Work out the finished part from the listing and answer in its coordinate system (mm). A direction names the side the tool comes from. Coordinates: 2 decimals unless noted, no trailing zeros. Order: outer loops, then holes, each group sorted by start corner. A loop starts at its lowest first (then second) coordinate and runs counter-clockwise, first axis right, second up. Notation, with made-up numbers: M 3.5,0.5 L 39.5,0.5 A37 ccw 39.5,37.5 Z; hole C 72.5,-3 d7. An arc over 180 degrees is marked long. Use a Markdown table: item, result.
from build123d import *

# Parameters (mm, degrees)
SKETCH1_W                      = 15.75
SKETCH1_H                      = 21.4
BOSS_EXTRUDE1_DEPTH            = 12.7
SKETCH3_W                      = 0.75
SKETCH3_H                      = 4
SKETCH4_W                      = 0.75
SKETCH4_H                      = 4
SKETCH5_W                      = 0.75
SKETCH5_H                      = 4
SKETCH6_W                      = 0.75
SKETCH6_H                      = 4
SKETCH7_W                      = 0.75
SKETCH7_H                      = 4
SKETCH8_W                      = 0.75
SKETCH8_H                      = 4
SKETCH9_W                      = 1.5
SKETCH9_H                      = 2
SKETCH10_W                     = 1
SKETCH10_H                     = 2
SKETCH11_W                     = 1
SKETCH11_H                     = 2
F_6_5_6_5_DIAMETER_HOLE1_D     = 6.5
F_6_5_6_5_DIAMETER_HOLE1_DEPTH = 30.123611625
F_6_5_6_5_DIAMETER_HOLE1_TIP   = 1.876388375
FILLET1_R                      = 0.3
FILLET2_R                      = 0.5


with BuildPart() as part:
    # Sketch1 → Boss-Extrude1 (new body)
    with BuildSketch(Plane.XZ):
        with Locations((1.445, -10.7)):
            Rectangle(SKETCH1_W, SKETCH1_H)
    extrude(amount=-BOSS_EXTRUDE1_DEPTH)

    # Sketch2 → Revolve1 (revolve)
    with BuildSketch(Plane.XZ.offset(-6.5)):
        Polygon((4.15, -21.4), (0, -21.4), (0, -24.3), (3.5, -24.3), align=None)
    revolve(axis=Axis((0, 6.5, -21.4), (0, 0, -1)))

    # Sketch3 → Contact Pin #1 (revolve)
    with BuildSketch(Plane.XY.offset(-10.6)):
        with Locations((-3.825, -2)):
            Rectangle(SKETCH3_W, SKETCH3_H)
    revolve(axis=Axis((-4.2, 0, -10.6), (0, -1, 0)))

    # Sketch4 → Contact Pin #2 (revolve)
    with BuildSketch(Plane.XY.offset(-10.6)):
        with Locations((7.605, -2)):
            Rectangle(SKETCH4_W, SKETCH4_H)
    revolve(axis=Axis((7.23, 0, -10.6), (0, -1, 0)))

    # Sketch5 → Contact Pin #3 (revolve)
    with BuildSketch(Plane.XY.offset(-16.95)):
        with Locations((-3.825, -2)):
            Rectangle(SKETCH5_W, SKETCH5_H)
    revolve(axis=Axis((-4.2, 0, -16.95), (0, -1, 0)))

    # Sketch6 → Contact Pin #4 (revolve)
    with BuildSketch(Plane.XY.offset(-4.25)):
        with Locations((-3.825, -2)):
            Rectangle(SKETCH6_W, SKETCH6_H)
    revolve(axis=Axis((-4.2, 0, -4.25), (0, -1, 0)))

    # Sketch7 → Contact Pin #5 (revolve)
    with BuildSketch(Plane.XY.offset(-16.95)):
        with Locations((7.605, -2)):
            Rectangle(SKETCH7_W, SKETCH7_H)
    revolve(axis=Axis((7.23, 0, -16.95), (0, -1, 0)))

    # Sketch8 → Contact Pin #6 (revolve)
    with BuildSketch(Plane.XY.offset(-4.25)):
        with Locations((7.605, -2)):
            Rectangle(SKETCH8_W, SKETCH8_H)
    revolve(axis=Axis((7.23, 0, -4.25), (0, -1, 0)))

    # Sketch9 → Revolve8 (revolve)
    with BuildSketch(Plane.XY.offset(-13.8)):
        with Locations((5.85, -1)):
            Rectangle(SKETCH9_W, SKETCH9_H)
    revolve(axis=Axis((5.1, 0, -13.8), (0, -1, 0)))

    # Sketch10 → Revolve9 (revolve)
    with BuildSketch(Plane.XY.offset(-7.45)):
        with Locations((7.73, -1)):
            Rectangle(SKETCH10_W, SKETCH10_H)
    revolve(axis=Axis((7.23, 0, -7.45), (0, -1, 0)))

    # Sketch11 → Revolve10 (revolve)
    with BuildSketch(Plane.XY.offset(-7.45)):
        with Locations((-3.7, -1)):
            Rectangle(SKETCH11_W, SKETCH11_H)
    revolve(axis=Axis((-4.2, 0, -7.45), (0, -1, 0)))

    # Sketch12 → Revolve11 (revolve)
    with BuildSketch(Plane.XZ.offset(-6.5)):
        Polygon((4.45, 8.9), (0, 8.9), (0, 0), (5.6, 0), (5.6, 3.83604719), (4.45, 4.5), align=None)
    revolve(axis=Axis((0, 6.5, 8.9), (0, 0, -1)))

    # Ø6.5 (6.5) Diameter Hole1
    with Locations(Plane.XY.offset(8.9)):
        with Locations((0, 6.5)):
            Hole(F_6_5_6_5_DIAMETER_HOLE1_D / 2, depth=F_6_5_6_5_DIAMETER_HOLE1_DEPTH)
            with Locations((0, 0, -(F_6_5_6_5_DIAMETER_HOLE1_DEPTH + F_6_5_6_5_DIAMETER_HOLE1_TIP / 2))):  # 120° drill point
                Cone(0, F_6_5_6_5_DIAMETER_HOLE1_D / 2, F_6_5_6_5_DIAMETER_HOLE1_TIP, mode=Mode.SUBTRACT)

    # Fillet1
    fillet1_edges = [part.edges().sort_by_distance(p)[0] for p in [
        (-4.45, 6.5, 8.9),
    ]]
    fillet(fillet1_edges, radius=FILLET1_R)

    # Fillet2
    fillet2_edges = [part.edges().sort_by_distance(p)[0] for p in [
        (3.25, 6.5, 8.9),
    ]]
    fillet(fillet2_edges, radius=FILLET2_R)


solid = part.part
1. Section D-D on x = 7.23 is taken. Determine the outline of the cut face in (y, z).
Answers below:
| item | result |
|---|---|
| outline | M -4,-17.7 L 0,-17.7 L 0,-21.4 L 12.7,-21.4 L 12.7,0 L 0,0 L 0,-3.5 L -4,-3.5 L -4,-5 L 0,-5 L 0,-6.45 L -2,-6.45 L -2,-8.45 L 0,-8.45 L 0,-9.85 L -4,-9.85 L -4,-11.35 L 0,-11.35 L 0,-16.2 L -4,-16.2 Z |
2. For faces 1 (the face through (-4, -2, -7)), 2 (the face through (-3.51, -1.97, -17.24)), 3 (the face through (3, 3, -21.4)), determine the directions among +Z, -Z, +X, -X, +Y, -Y from which every point of the face is accessible in a straight line to the end or side of a thin tool.
Answers below:
| item | result |
|---|---|
| face 1 | +X, -X, -Y |
| face 2 | -Y |
| face 3 | -Z |
3. Find the intervals of material crossed by probe 1 along Y at (x, z) = (0, -7); probe 2 along Y at (x, z) = (0, 0.5); probe 3 along X at (y, z) = (6.5, -5), in increasing order.
Answers below:
| item | result |
|---|---|
| probe 1 | 0 to 3.25, 9.75 to 12.7 |
| probe 2 | 0.9 to 3.25, 9.75 to 12.1 |
| probe 3 | -6.43 to -3.25, 3.25 to 9.32 |
4. Flat-ended cylindrical pins translate along their axes: P1, Ø6, axis at x = -3.5, y = 10, coming from the -Z side; P2, Ø8, axis at x = -4, z = 3.5, coming from the -Y side; P3, Ø6, axis at x = 6, y = 0.5, coming from the +Z side; P4, Ø2, axis at x = 7, z = -7.5, coming from the -Y side. Find the tip coordinate at first contact, or state that the pin passes through.
Answers below:
| item | result |
|---|---|
| P1 | z = -24.3 |
| P2 | y = 0 |
| P3 | z = 3.9 |
| P4 | y = -2 |
5. Section B-B on z = -13.8 is taken. Determine the outline of the cut face in (x, y).
Answers below:
| item | result |
|---|---|
| outline | M -6.43,0 L 3.6,0 L 3.6,-2 L 6.6,-2 L 6.6,0 L 9.32,0 L 9.32,12.7 L -6.43,12.7 Z; hole C 0,6.5 d6.5 |
6. Section A-A on y = -1 is taken. Give the number of separate pieces and of enclosed holes in the cut face, then the cut area to 3 significant figures.
Answers below:
| item | result |
|---|---|
| separate pieces | 9 |
| enclosed holes | 0 |
| area | 24.0 mm² |
7. For a pull along Z with two mould halves and no side action, classify faces 4 (the face through (7.067, -1.972, -11.332)), 5 (the face through (7, -4, -4)), 6 (the face through (0, 6, -24.3)) as +Z half, -Z half, draft (parallel to the pull), parting line (faces both ways), or undercut.
Answers below:
| item | result |
|---|---|
| face 4 | undercut |
| face 5 | draft |
| face 6 | -Z half |
8. Section C-C on z = -7.45 is taken. Determine the outline of the cut face in (x, y), then the cut area to 3 significant figures.
Answers below:
| item | result |
|---|---|
| outline | M -6.43,0 L -5.2,0 L -5.2,-2 L -3.2,-2 L -3.2,0 L 6.23,0 L 6.23,-2 L 8.23,-2 L 8.23,0 L 9.32,0 L 9.32,12.7 L -6.43,12.7 Z; hole C 0,6.5 d6.5 |
| area | 175 mm² |
